Input: part model. Units: mm. Frame: model coordinates. Coordinates: 2 decimals unless noted, no trailing zeros. Order: outer loops, then holes, each group sorted by start corner. A loop starts at its lowest first (then second) coordinate and runs counter-clockwise, first axis right, second up. Notation, with made-up numbers: M -1.75,-33.75 L 18.25,-33.75 A38 cw 18.25,4.25 Z; hole C -13,77 d1. An arc over 180 degrees is marked long. Answer in a Markdown table with one row per item.
Autodesk Inventor part; units mm, degrees
ref_plane "YZ Plane" through (0, 0, 0) normal (1, 0, 0) x (0, 1, 0)
ref_plane "XZ Plane" through (0, 0, 0) normal (0, 1, 0) x (-1, 0, 0)
ref_plane "XY Plane" through (0, 0, 0) normal (0, 0, 1) x (1, 0, 0)
sketch "スケッチ1" plane through (0, 0, 0) normal (0, 0, 1) x (1, 0, 0)
  circle A0 centre (0, 0) radius 52.5 construction
  circle A1 centre (0, 0) radius 12.55 construction
  circle A2 centre (-12.3744, 12.3744) radius 2.05 construction
  circle A3 centre (-12.3744, -12.3744) radius 2.05 construction
  circle A4 centre (12.3744, -12.3744) radius 2.05 construction
  circle A5 centre (12.3744, 12.3744) radius 2.05 construction
  line L0 (0, 0) -> (-12.3744, 12.3744) construction
  line L1 (0, 0) -> (0, 12.55) construction
  circle A6 centre (0, 0) radius 23.5 construction
  line L2 (-52.5, 39.5) -> (52.5, 39.5)
  line L3 (52.5, 39.5) -> (52.5, -24.4454)
  line L4 (52.5, -24.4454) -> (-52.5, -24.4454)
  line L5 (-52.5, -24.4454) -> (-52.5, 39.5)
  line L6 (-52.5, 24.5) -> (52.5, 24.5) construction
  line L7 (-52.5, 32) -> (52.5, 32) construction
  circle A7 centre (0, 32) radius 1.55
  circle A8 centre (-45, 32) radius 1.55
  circle A9 centre (45, 32) radius 1.55
  circle A10 centre (-19.4454, 19.4454) radius 1.55 construction
  circle A11 centre (-19.4454, -19.4454) radius 1.55 construction
  circle A12 centre (19.4454, -19.4454) radius 1.55 construction
  circle A13 centre (19.4454, 19.4454) radius 1.55 construction
  circle A14 centre (0, 0) radius 16.05
  circle A15 centre (-55.5, -20.4454) radius 1.5
  line L8 (-52.5, -24.4454) -> (-55.5, -24.4454)
  arc A16 (-55.5, -16.4454) -> (-55.5, -24.4454) centre (-55.5, -20.4454) ccw
  line L9 (-55.5, -16.4454) -> (-52.5, -16.4454)
  circle A17 centre (55.5, -20.4454) radius 1.5
  line L10 (52.5, -24.4454) -> (55.5, -24.4454)
  arc A18 (55.5, -24.4454) -> (55.5, -16.4454) centre (55.5, -20.4454) ccw
  line L11 (55.5, -16.4454) -> (52.5, -16.4454)
  point P0 (0, 39.5)
  point P1 (0, 23.5)
  point P2 (0, -52.5)
  dimension "d0" = 105
  dimension "d1" = 25.1
  dimension "d9" = 47
  dimension "d2" = 4.1
  dimension "d5" = 360
  dimension "d7" = 45
  dimension "d8" = 35
  dimension "d10" = 15
  dimension "d18" = 105
  dimension "d20" = 7.5
  dimension "d21" = 3.1
  dimension "d22" = 3.1
  dimension "d23" = 3.1
  dimension "d24" = 90
  dimension "d27" = 3.1
  dimension "d30" = 360
  dimension "d32" = 55
  dimension "d33" = 32.1
  dimension "d41" = 5
  dimension "d42" = 3
  dimension "d43" = 4
  dimension "d44" = 3
  dimension "d45" = 92
extrude "押し出し1" add sketch "スケッチ1" along normal blind 2
sketch "スケッチ2" plane through (0, 0, 2) normal (0, 0, 1) x (1, 0, 0)
  line L0 (-22.86, -0.3048) -> (22.86, -0.3048) construction
  line L1 (0, -0.3048) -> (0, 0) construction
  circle A0 centre (-22.86, -0.3048) radius 1.55
  circle A1 centre (22.86, -0.3048) radius 1.55
  line L2 (0, 0) -> (0, 0.3048) construction
  dimension "d34" = 0.3048
  dimension "d35" = 45.72
  dimension "d36" = 3.1
  dimension "d37" = 3.1
  dimension "d40" = 0.3048
extrude "押し出し2" cut sketch "スケッチ2" against normal through all
fillet "フィレット1" radius 5 4 edges at (-52.5, -16.4454, 1) (-52.5, 39.5, 1) (52.5, 39.5, 1) (52.5, -16.4454, 1)
sketch "スケッチ3" plane through (0, 0, 2) normal (0, 0, 1) x (1, 0, 0)
  arc A0 (52.5, 34.5) -> (47.5, 39.5) centre (47.5, 34.5) ccw
  line L0 (47.5, 39.5) -> (-47.5, 39.5)
  arc A1 (-47.5, 39.5) -> (-52.5, 34.5) centre (-47.5, 34.5) ccw
  line L1 (-52.5, 34.5) -> (-52.5, -11.6705)
  arc A2 (-56.3889, -16.5455) -> (-52.5, -11.6705) centre (-57.5, -11.6705) ccw
  arc A3 (-56.3889, -16.5455) -> (-55.5, -24.4454) centre (-55.5, -20.4454) ccw
  line L2 (-55.5, -24.4454) -> (55.5, -24.4454)
  arc A4 (55.5, -24.4454) -> (56.3889, -16.5455) centre (55.5, -20.4454) ccw
  arc A5 (52.5, -11.6705) -> (56.3889, -16.5455) centre (57.5, -11.6705) ccw
  line L3 (52.5, -11.6705) -> (52.5, 34.5)
  circle A6 centre (22.86, -0.3048) radius 1.55
  circle A7 centre (-22.86, -0.3048) radius 1.55
  circle A8 centre (0, 32) radius 1.55
  circle A9 centre (-45, 32) radius 1.55
  circle A10 centre (45, 32) radius 1.55
  circle A11 centre (0, 0) radius 16.05
  circle A12 centre (55.5, -20.4454) radius 1.5
  circle A13 centre (-55.5, -20.4454) radius 1.5
equation "\"d20\" = 0.5 * d10"
equation "\"d40\" = d34"
properties part number "omu_al_jo_3" material "アルミニウム 6061-AHC"
1) Cut plane D-D, the plane z = 0.9. State how many separate pieces and enclosed holes the cut face has, and give its area (3 significant figures).
Resolved:
| item | result |
|---|---|
| separate pieces | 1 |
| enclosed holes | 8 |
| area | 5,950 mm2 |
2) Cut plane A-A, the plane x = 45. Output: boundary loops of the cut face in (y, z), and give its area (3 significant figures).
Resolved:
| item | result |
|---|---|
| outline | M -24.45,0 L 30.45,0 L 30.45,2 L -24.45,2 Z; M 33.55,0 L 39.5,0 L 39.5,2 L 33.55,2 Z |
| area | 122 mm2 |
3) Cut plane C-C, the plane y = 14. Output: boundary loops of the cut face in (x, z), and give its area (3 significant figures).
Resolved:
| item | result |
|---|---|
| outline | M -52.5,0 L -7.85,0 L -7.85,2 L -52.5,2 Z; M 7.85,0 L 52.5,0 L 52.5,2 L 7.85,2 Z |
| area | 179 mm2 |
4) Material intervals for probe 1 along Y at (x, z) = (0, 0.6); probe 2 along Y at (x, z) = (-45, 1.5); probe 3 along X at (y, z) = (0.5, 1.9), sorted ascending.
Resolved:
| item | result |
|---|---|
| probe 1 | y = -24.45 to -16.05, 16.05 to 30.45, 33.55 to 39.5 |
| probe 2 | y = -24.45 to 30.45, 33.55 to 39.5 |
| probe 3 | x = -52.5 to -24.18, -21.54 to -16.04, 16.04 to 21.54, 24.18 to 52.5 |
5) Cut plane B-B, the plane y = 32. Output: boundary loops of the cut face in (x, z).
Resolved:
| item | result |
|---|---|
| outline | M -52.5,0 L -46.55,0 L -46.55,2 L -52.5,2 Z; M -43.45,0 L -1.55,0 L -1.55,2 L -43.45,2 Z; M 1.55,0 L 43.45,0 L 43.45,2 L 1.55,2 Z; M 46.55,0 L 52.5,0 L 52.5,2 L 46.55,2 Z |
6) Contact query for flat-ended pins moving along their axis: pin 1 (4 mm diameter, centred on x = 0, y = 32, fed in from -Z); pin 2 (2.5 mm diameter, centred on x = 45, y = 32, fed in from -Z). Output: stop coordinate, or through.
Resolved:
| item | result |
|---|---|
| pin 1 | stops at z = 0 |
| pin 2 | passes through |
7) Mould query, pull axis X, two halves, no side actions, for faces 1 (the face through (59.483, -20.811, 0.986)), 2 (the face through (-51, 38.07, 1.01)), 3 (the face through (-0.202, 30.463, 0.986)). Classes: +X half, -X half, draft (parallel to the pull), parting line (faces both ways), or undercut.
Resolved:
| item | result |
|---|---|
| face 1 | +X half |
| face 2 | -X half |
| face 3 | undercut |
